Input: part model. Units: mm. Frame: model coordinates. A direction names the side the tool comes from. Give positions to 0.01 mm unless a question says otherwise; leave off trailing zeros. Loops run counter-clockwise (first coordinate to the right, second up) from the corner with the lowest first, then second, coordinate; pieces in that order, holes last.
from build123d import *

# Parameters (mm, degrees)
SKETCH1_W           = 80
SKETCH1_H           = 60
SKETCH1_R           = 1.5
SKETCH1_R_2         = 2
SKETCH1_W_2         = 13.5
SKETCH1_H_2         = 20.585457955
SKETCH1_W_3         = 28.5
SKETCH1_W_4         = 8
BOSS_EXTRUDE1_DEPTH = 3


with BuildPart() as part:
    # Sketch1 → Boss-Extrude1 (new body)
    with BuildSketch(Plane.XY):
        Rectangle(SKETCH1_W, SKETCH1_H)
        with Locations((-37, 27)):
            Circle(SKETCH1_R, mode=Mode.SUBTRACT)
        with Locations(Location((-37, -27, 0), (0, 0, 180))):
            Circle(SKETCH1_R, mode=Mode.SUBTRACT)
        with Locations((37, -27)):
            Circle(SKETCH1_R, mode=Mode.SUBTRACT)
        with Locations(Location((37, 27, 0), (0, 0, 180))):
            Circle(SKETCH1_R, mode=Mode.SUBTRACT)
        with Locations((32.5, 0)):
            Circle(SKETCH1_R_2, mode=Mode.SUBTRACT)
        with Locations((12.5, 0)):
            Circle(SKETCH1_R_2, mode=Mode.SUBTRACT)
        with Locations((-22.5, 0)):
            Circle(SKETCH1_R_2, mode=Mode.SUBTRACT)
        with Locations((22.5, -13.457271023)):
            Rectangle(SKETCH1_W_2, SKETCH1_H_2, mode=Mode.SUBTRACT)
        with Locations((-5, 13.457271023)):
            Rectangle(SKETCH1_W_3, SKETCH1_H_2, mode=Mode.SUBTRACT)
        with Locations((22.5, 13.457271023)):
            Rectangle(SKETCH1_W_2, SKETCH1_H_2, mode=Mode.SUBTRACT)
        with Locations((-29.75, 13.457271023)):
            Rectangle(SKETCH1_W_4, SKETCH1_H_2, mode=Mode.SUBTRACT)
        with Locations((-5, -13.457271023)):
            Rectangle(SKETCH1_W_3, SKETCH1_H_2, mode=Mode.SUBTRACT)
        with Locations((-29.75, -13.457271023)):
            Rectangle(SKETCH1_W_4, SKETCH1_H_2, mode=Mode.SUBTRACT)
    extrude(amount=BOSS_EXTRUDE1_DEPTH)


solid = part.part
(1) Mould query, pull axis X, two halves, no side actions, for faces 1 (the cylindrical face through (-24.1, -1.2, 1.5)), 2 (the flat face through (-40, 0, 1)), 3 (the flat face through (-1, -30, 1)). Classes: +X half, -X half, draft (parallel to the pull), parting line (faces both ways), or undercut.
Values follow:
face 1: undercut
face 2: -X half
face 3: draft
(2) Ray query, probe 1 along X at (y, z) = (-16, 0.3); probe 2 along Y at (x, z) = (37, 1.6); probe 3 along Y at (x, z) = (28, 2.05). Return the intervals inside material, ascending.
Values follow:
probe 1: x = -40 to -33.75, -25.75 to -19.25, 9.25 to 15.75, 29.25 to 40
probe 2: y = -30 to -28.5, -25.5 to 25.5, 28.5 to 30
probe 3: y = -30 to -23.75, -3.16 to 3.16, 23.75 to 30
(3) Cut plane B-B (x = -37). Return the cut outline in (y, z), and give its area (3 significant figures).
Values follow:
outline: (-30, 0) - (-28.5, 0) - (-28.5, 3) - (-30, 3) - close; (-25.5, 0) - (25.5, 0) - (25.5, 3) - (-25.5, 3) - close; (28.5, 0) - (30, 0) - (30, 3) - (28.5, 3) - close
area: 162 mm2
(4) Cut plane D-D (y = 11). Return the cut outline in (x, z).
Values follow:
outline: (-40, 0) - (-33.75, 0) - (-33.75, 3) - (-40, 3) - close; (-25.75, 0) - (-19.25, 0) - (-19.25, 3) - (-25.75, 3) - close; (9.25, 0) - (15.75, 0) - (15.75, 3) - (9.25, 3) - close; (29.25, 0) - (40, 0) - (40, 3) - (29.25, 3) - close
(5) Reachability of faces 4 (the flat face through (29.25, 13, 1)), 5 (the flat face through (-1, 0, 3)) from +Z, -Z, +X, -X, +Y, -Y: full face, straight path, thin tool, end or side. Return the list, or none.
Values follow:
face 4: +Z, -Z
face 5: +Z, +X, -X, +Y, -Y
(6) Cut plane A-A (y = 27). Return the cut outline in (x, z).
Values follow:
outline: (-40, 0) - (-38.5, 0) - (-38.5, 3) - (-40, 3) - close; (-35.5, 0) - (35.5, 0) - (35.5, 3) - (-35.5, 3) - close; (38.5, 0) - (40, 0) - (40, 3) - (38.5, 3) - close
(7) Pin query (flat end, axial travel): pin 1 Ø10 at (x, y) = (26.5, 17.5) entering from -Z. Return the tip coordinate at first contact, or that it passes through.
Values follow:
pin 1: stops at z = 0
(8) Cut plane C-C (x = 12.5). Return the cut outline in (y, z).
Values follow:
outline: (-30, 0) - (-2, 0) - (-2, 3) - (-30, 3) - close; (2, 0) - (30, 0) - (30, 3) - (2, 3) - close
